The model under review builds one solid part; all positions refer to its coordinate system, in mm. A direction names the side the tool comes from. Give positions to 0.01 mm unless a question says otherwise; leave off trailing zeros. Write each loop counter-clockwise with the first axis right and the second up, starting at its lowest first coordinate (ties: lowest second). Pieces come first, ordered by that corner, then holes. Notation, with made-up numbers: M -13.75,81 L 43.25,81 A27 ccw 43.25,97 Z; hole C -19.5,10 d6. An arc over 180 degrees is marked long. Write item = value, one per line. Start each with the question number.
```python
from build123d import *

# Parameters (mm, degrees)
BOX_W                    = 13.22
BOX_H                    = 13.22
BOX_DEPTH                = 40
CYLINDER_R               = 9.35
CYLINDER_DEPTH           = 25
CYLINDER_PLACEMENT_ANGLE = 315
SKETCH_R                 = 1.5
POCKET_DEPTH             = 2.741
POCKET_DEPTH_BACK        = 15.961


with BuildPart() as cube:
    # Box → Box (new body)
    with BuildSketch(Plane.XY):
        with Locations((6.61, 6.61)):
            Rectangle(BOX_W, BOX_H)
    extrude(amount=BOX_DEPTH)


with BuildPart() as body:
    # Cylinder → Cylinder (new body)
    with BuildSketch(Plane.XY):
        Circle(CYLINDER_R)
    extrude(amount=CYLINDER_DEPTH)


with BuildPart() as body_1:
    # Cylinder placement: moved
    add(body.part.moved(Location((6.61, 6.61, 0))).rotate(Axis((6.61, 6.61, 0), (0, 0, 1)), CYLINDER_PLACEMENT_ANGLE))

    # Fusion: union Cube
    add(cube.part)

    # Sketch (on Face6 of Fusion) → Pocket (cut, two sides)
    with BuildSketch(Plane(origin=(0, 13.22, 0), x_dir=(-1, 0, 0), z_dir=(0, 1, 0))) as pocket_sk:
        with Locations((-6.61, 20)):
            Circle(SKETCH_R)
    extrude(amount=POCKET_DEPTH, mode=Mode.SUBTRACT)
    extrude(pocket_sk.sketch, amount=-POCKET_DEPTH_BACK, mode=Mode.SUBTRACT)


solid = body_1.part
```
Item 1: We need section D-D, the plane y = 1. Write out the cut boundary in (x, z).
Item 2: Clearance check with flat-ended pins moving along their axes: P1, Ø10.5, axis at x = 6, z = 32, coming from the +Y side; P2, Ø5, axis at y = 6.5, z = 29.5, coming from the -X side; P3, Ø1.8, axis at x = 6.61, z = 20, coming from the +Y side; P4, Ø6, axis at y = -0.5, z = 35, coming from the +X side. State where each tip first meets the part, or that it passes through.
Item 3: To check wall thickness, follow probe 1 along Z at (x, y) = (6.61, 10); probe 2 along Y at (x, z) = (9.5, 30); probe 3 along Z at (x, y) = (-0.25, 6.5). State the ranges of each line that lie inside material, in increasing order. Write a range as [from, to].
Item 4: We need section C-C, the plane z = 20. Write out the cut boundary in (x, y), and give its area (3 significant figures).
Item 5: We need section B-B, the plane y = 6.61. Write out the cut boundary in (x, z), and give its area (3 significant figures).
Item 6: We need section A-A, the plane x = 6.61. Write out the cut boundary in (y, z), and give its area (3 significant figures).
Item 7: The part is to be moulded in two halves that separate along X. For faces 1 (the flat face through (0, 7, 32)), 2 (the cylindrical face through (6.805, 6.741, 21.487)), 3 (the flat face through (7, 7, 40)), 4 (the cylindrical face through (3.795, -2.306, 12.325)), say which applies: released by +X, released by -X, zero draft, split by the parting line, or undercut.
Item 8: For faces 5 (the flat face through (6, 7, 0)), 6 (the flat face through (7, 0, 32)), 7 (the flat face through (5.6, -0.2, 25)), 8 (the flat face through (7, 13.22, 32)), 9 (the flat face through (13.22, 7, 32)), list the 3-axis set-ups (+Z, -Z, +X, -X, +Y, -Y) from which the entire face can be reached by the end or side of a thin tool; tool diameter is ignored.
Worked out:
q1.outline = M -0.87,0 L 14.09,0 L 14.09,25 L 13.22,25 L 13.22,40 L 0,40 L 0,25 L -0.87,25 Z; hole C 6.61,20 d3
q2.P1 = 13.22
q2.P2 = 0
q2.P3 = through
q2.P4 = 13.22
q3.probe_1 = [0, 18.5], [21.5, 40]
q3.probe_2 = [0, 13.22]
q3.probe_3 = [0, 25]
q4.outline = M 5.11,-2.62 L 5.11,15.84 A9.35 ccw Z; M 8.11,-2.62 A9.35 ccw 8.11,15.84 Z
q4.area = 219 mm²
q5.outline = M -2.74,0 L 15.96,0 L 15.96,25 L 13.22,25 L 13.22,40 L 0,40 L 0,25 L -2.74,25 Z; hole C 6.61,20 d3
q5.area = 659 mm²
q6.outline = M -2.74,0 L 15.96,0 L 15.96,18.5 L -2.74,18.5 Z; M -2.74,21.5 L 15.96,21.5 L 15.96,25 L 13.22,25 L 13.22,40 L 0,40 L 0,25 L -2.74,25 Z
q6.area = 610 mm²
q7.face_1 = released by -X
q7.face_2 = undercut
q7.face_3 = zero draft
q7.face_4 = split by the parting line
q8.face_5 = -Z, +X, -X, +Y, -Y
q8.face_6 = +Z, +X, -X, -Y
q8.face_7 = +Z
q8.face_8 = +Z, +X, -X, +Y
q8.face_9 = +Z, +X, +Y, -Y
